from build123d import *

# Parameters (mm, degrees)
F0_R     = 15
F1_DEPTH = 76.2
F2_R     = 5.08
F3_R     = 12.46
F4_DEPTH = 76.201


with BuildPart() as f1:
    # F0 (on Top) → F1 (new body)
    with BuildSketch(Plane.XY):
        Circle(F0_R)
    extrude(amount=F1_DEPTH)

    # F2
    f2_edges = [f1.edges().sort_by_distance(p)[0] for p in [
        (-15, 0, 0),
    ]]
    fillet(f2_edges, radius=F2_R)

    # F3 (on face) → F4 (cut, through all)
    with BuildSketch(Plane.XY.offset(76.2)):
        Circle(F3_R)
    extrude(amount=-F4_DEPTH, mode=Mode.SUBTRACT)


solid = f1.part
Geometry: final body of the model. Coordinates: model frame, mm. Give positions to 0.01 mm unless a question says otherwise; leave off trailing zeros. Write each loop counter-clockwise with the first axis right and the second up, starting at its lowest first coordinate (ties: lowest second). Pieces come first, ordered by that corner, then holes.
(1) Cut plane C-C, the plane z = 59.5. Return loops of the section in (x, y).
(2) Mould query, pull axis Y, two halves, no side actions, for faces 1 (the flat face through (-3.4, 12.3, 76.2)), 2 (the cylindrical face through (-14.985, 0.66, 40.142)), 3 (the cylindrical face through (11.9, 3.7, 39)). Classes: released by +Y, released by -Y, zero draft, split by the parting line, or undercut.
(3) Cut plane A-A, the plane x = 0. Return loops of the section in (y, z), then the cut area to 3 significant figures.
(4) Ray query, line 1 (Y direction, x = 0, z = 27); line 2 (Y direction, x = -1.25, z = 28); line 3 (X direction, y = 2.75, z = 32). Return the intervals inside material, ascending.
(5) First-contact query: P1, Ø2, axis at y = -8.5, z = 26, coming from the +X side; P2, Ø2, axis at y = 11.5, z = 46.5, coming from the -X side; P3, Ø1, axis at y = -11.5, z = 64, coming from the +X side. Flat tips, straight axial feed; report the tip coordinate or a pass-through.
Values follow:
1. outline: circle Ø30 at (0, 0); hole circle Ø24.92 at (0, 0)
2. face 1: zero draft
2. face 2: split by the parting line
2. face 3: undercut
3. outline: (-15, 5.08) arc R5.08 ccw to (-12.46, 0.68) - (-12.46, 76.2) - (-15, 76.2) - close; (12.46, 0.68) arc R5.08 ccw to (15, 5.08) - (15, 76.2) - (12.46, 76.2) - close
3. area: 377 mm2
4. line 1: y = -15 to -12.46, 12.46 to 15
4. line 2: y = -14.95 to -12.4, 12.4 to 14.95
4. line 3: x = -14.75 to -12.15, 12.15 to 14.75
5. P1: stops at x = 12.99
5. P2: stops at x = -10.71
5. P3: stops at x = 10.2
